from build123d import *

# Parameters (mm, degrees)
SKETCH1_R           = 21.15
SKETCH1_R_2         = 16.35319065
SKETCH1_R_3         = 13.728990349
SKETCH1_R_4         = 4.65
BOSS_EXTRUDE1_DEPTH = 1.5
SKETCH1_3_R         = 16.35319065
SKETCH1_3_R_2       = 13.728990349
BOSS_EXTRUDE2_DEPTH = 3.5


with BuildPart() as part:
    # Sketch1 → Boss-Extrude1 (new body)
    # profile 1 of 3: a face of its own
    with BuildSketch(Plane(origin=(0, 0, 0), x_dir=(1, 0, 0), z_dir=(0, 1, 0))):
        with Locations(Location((0, 0, 0), (0, 0, 270))):
            Circle(SKETCH1_R)
        Circle(SKETCH1_R_2, mode=Mode.SUBTRACT)
    # profile 2 of 3: a face of its own
    with BuildSketch(Plane(origin=(0, 0, 0), x_dir=(1, 0, 0), z_dir=(0, 1, 0))):
        Circle(SKETCH1_R_2)
        Circle(SKETCH1_R_3, mode=Mode.SUBTRACT)
    # profile 3 of 3: a face of its own
    with BuildSketch(Plane(origin=(0, 0, 0), x_dir=(1, 0, 0), z_dir=(0, 1, 0))):
        Circle(SKETCH1_R_3)
        with Locations(Location((0, 0, 0), (0, 0, 270))):
            Circle(SKETCH1_R_4, mode=Mode.SUBTRACT)
    extrude(amount=BOSS_EXTRUDE1_DEPTH)

    # Sketch1_3 → Boss-Extrude2 (add)
    with BuildSketch(Plane(origin=(0, 0, 0), x_dir=(1, 0, 0), z_dir=(0, 1, 0))):
        with Locations(Location((0, 0, 0), (0, 0, 270))):
            Circle(SKETCH1_3_R)
        with Locations(Location((0, 0, 0), (0, 0, 270))):
            Circle(SKETCH1_3_R_2, mode=Mode.SUBTRACT)
    extrude(amount=BOSS_EXTRUDE2_DEPTH)


solid = part.part
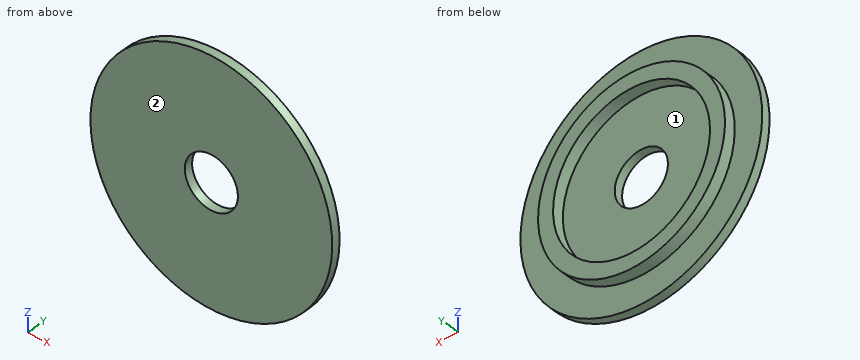
Geometry check sheet. Reference: the model listing, model coordinates, mm. Face numbers are marked on the shaded views. A direction names the side the tool comes from. Round coordinates to 2 decimals unless told otherwise and drop trailing zeros. Write each loop counter-clockwise with the first axis right and the second up, starting at its lowest first coordinate (ties: lowest second). Pieces come first, ordered by that corner, then holes.
Item 1: Section check D-D (z = 9.5). Record the boundary of the cut face in (x, y), plus the area to 3 significant figures.
Determined:
outline: (-18.9, 0) - (18.9, 0) - (18.9, 1.5) - (13.31, 1.5) - (13.31, 3.5) - (9.91, 3.5) - (9.91, 1.5) - (-9.91, 1.5) - (-9.91, 3.5) - (-13.31, 3.5) - (-13.31, 1.5) - (-18.9, 1.5) - close
area: 70.3 mm2
Item 2: Section check C-C (y = 2.7). Record the boundary of the cut face in (x, z), plus the area to 3 significant figures.
Determined:
outline: circle Ø32.71 at (0, 0); hole circle Ø27.46 at (0, 0)
area: 248 mm2
Item 3: Go/stop test with flat-tipped pins: pin 1 Ø2 at (x, z) = (-4, 15.5) entering from -Y; pin 2 Ø1.5 at (x, y) = (-16.5, 1) entering from +Z; pin 3 Ø1.5 at (x, z) = (-3.5, 5.5) entering from +Y; pin 4 Ø1 at (y, z) = (1, -14.5) entering from +X. Record where each tip stops, or that it passes through.
Determined:
pin 1: stops at y = 0
pin 2: stops at z = 14.12
pin 3: stops at y = 1.5
pin 4: stops at x = 15.85
Item 4: Access from +Z, -Z, +X, -X, +Y, -Y to the whole of each face (thin tool, end or side, straight path). Record for the marked faces 1 and 2.
Determined:
face 1: +Y
face 2: +Z, -Z, +X, -X, -Y
Item 5: Material ranges on line 1 along X through (y, z) = (0.4, 0); line 2 along X through (y, z) = (2.65, 0); line 3 along Y through (x, z) = (11, -1), recorded low to high.
Determined:
line 1: x = -21.15 to -4.65, 4.65 to 21.15
line 2: x = -16.35 to -13.73, 13.73 to 16.35
line 3: y = 0 to 1.5
Item 6: Section check A-A (x = 0). Record the boundary of the cut face in (y, z).
Determined:
outline: (0, -21.15) - (1.5, -21.15) - (1.5, -16.35) - (3.5, -16.35) - (3.5, -13.73) - (1.5, -13.73) - (1.5, -4.65) - (0, -4.65) - close; (0, 4.65) - (1.5, 4.65) - (1.5, 13.73) - (3.5, 13.73) - (3.5, 16.35) - (1.5, 16.35) - (1.5, 21.15) - (0, 21.15) - close
Item 7: Section check B-B (z = 0). Record the boundary of the cut face in (x, y), plus the area to 3 significant figures.
Determined:
outline: (-21.15, 0) - (-4.65, 0) - (-4.65, 1.5) - (-13.73, 1.5) - (-13.73, 3.5) - (-16.35, 3.5) - (-16.35, 1.5) - (-21.15, 1.5) - close; (4.65, 0) - (21.15, 0) - (21.15, 1.5) - (16.35, 1.5) - (16.35, 3.5) - (13.73, 3.5) - (13.73, 1.5) - (4.65, 1.5) - close
area: 60.0 mm2
